from build123d import *

# Parameters (mm, degrees)
SKETCH1_W           = 45
SKETCH1_H           = 45
SKETCH1_R           = 1.55
SKETCH1_R_2         = 3.75
SKETCH1_R_3         = 1.5
BOSS_EXTRUDE2_DEPTH = 3
CHAMFER1_SIZE       = 2
FILLET2_R           = 10


with BuildPart() as part:
    # Sketch1 → Boss-Extrude2 (new body)
    # profile 1 of 3: a face of its own
    with BuildSketch(Plane(origin=(0, 0, 0), x_dir=(0, 0, -1), z_dir=(1, 0, 0))):
        Polygon((0, 15), (27.5, 86.038878339), (39.282646226, 75.31968933), (11.439152216, 14.16907058), (50, 14.16907058), (82.089729195, 14.16907058), (77.753857358, 26.374167507), (66.036256754, 25.688126343), (64.741637437, 39.196033454), (73.198877763, 39.196033454), (60.365916003, 75.31968933), (72.5, 85.972228566), (97.712949054, 15), (100, 15), (100, 0), (75, 0), (75, 10), (72, 10), (72, 0), (28, 0), (28, 10), (25, 10), (25, 0), (0, 0), align=None)
        with BuildLine():
            Line((67.956429084, 33.345444875), (77.753857358, 33.345444875))
            ThreePointArc((77.753857358, 33.345444875), (79.253857358, 31.845444875), (77.753857358, 30.345444875))
            Line((77.753857358, 30.345444875), (67.956429084, 30.345444875))
            ThreePointArc((67.956429084, 30.345444875), (66.456429084, 31.845444875), (67.956429084, 33.345444875))
        make_face(mode=Mode.SUBTRACT)
    # profile 2 of 3: a face of its own
    with BuildSketch(Plane(origin=(0, 0, 0), x_dir=(0, 0, -1), z_dir=(1, 0, 0))):
        with Locations((50, 97.81968933)):
            Rectangle(SKETCH1_W, SKETCH1_H)
        with Locations((34.5, 82.31968933)):
            Circle(SKETCH1_R, mode=Mode.SUBTRACT)
        with Locations((65.5, 82.31968933)):
            Circle(SKETCH1_R, mode=Mode.SUBTRACT)
        with Locations((65.5, 113.31968933)):
            Circle(SKETCH1_R, mode=Mode.SUBTRACT)
        with Locations((34.5, 113.31968933)):
            Circle(SKETCH1_R, mode=Mode.SUBTRACT)
        with Locations((50, 97.81968933)):
            Circle(SKETCH1_R_2, mode=Mode.SUBTRACT)
    # profile 3 of 3: a face of its own
    with BuildSketch(Plane(origin=(0, 0, 0), x_dir=(0, 0, -1), z_dir=(1, 0, 0))):
        Polygon((58.527688318, 120.31968933), (90.14613276, 143.005488448), (95.440133744, 135.626948458), (68.383623973, 116.214274737), align=None)
        with Locations((89.319967142, 136.74442097)):
            Circle(SKETCH1_R_3, mode=Mode.SUBTRACT)
    extrude(amount=BOSS_EXTRUDE2_DEPTH)

    # Chamfer1
    chamfer1_edges = [part.edges().sort_by_distance(p)[0] for p in [
        (3, 82.31968933, -32.95),
        (3, 113.31968933, -32.95),
        (3, 113.31968933, -63.95),
        (3, 82.31968933, -63.95),
    ]]
    chamfer(chamfer1_edges, length=CHAMFER1_SIZE)

    # Fillet2
    fillet2_edges = [part.edges().sort_by_distance(p)[0] for p in [
        (1.5, 86.038878339, -27.5),
        (1.5, 75.31968933, -60.365916003),
        (1.5, 75.31968933, -39.282646226),
    ]]
    fillet(fillet2_edges, radius=FILLET2_R)


solid = part.part
Here's how the part is built. I have some questions about the finished solid (model axes, mm). A direction names the side the tool comes from. Coordinates: 2 decimals unless noted, no trailing zeros. Order: outer loops, then holes, each group sorted by start corner. A loop starts at its lowest first (then second) coordinate and runs counter-clockwise, first axis right, second up. Notation, with made-up numbers: (72, 15.5) - (104, 15.5) arc R3 ccw to (104, 20.5) - close; hole circle Ø7 at (56, 34). An arc over 180 degrees is marked (long way). Use CSV: the item, a comma, the result in double quotes. Start each with the question number.
1. For faces 4 (the face through (3, 73, -62)), 5 (the face through (1, 5, -72)), 6 (the face through (1, 30.345, -73)), which set-ups out of +Z, -Z, +X, -X, +Y, -Y let a thin tool reach every point of the face, with its end or its side?
2. Suppose I cut it at B-B on y = 55.5. List the corners of the cut face in (x, z) for me, then the cut area to 3 significant figures.
3. Suppose I cut it at A-A on z = -50. List the corners of the cut face in (x, y) for me, then the cut area to 3 significant figures.
4. Suppose I cut it at D-D on z = -34.5. List the corners of the cut face in (x, y) for me, then the cut area to 3 significant figures.
5. If we mould it in two halves opening along Y, with no side actions, what happens to faces 1 (the face through (1, 10, -27)), 2 (the face through (1, 102, -72.5)), 3 (the face through (0, 73, -62))? For each: +Y half, -Y half, draft (parallel to the pull), parting line (faces both ways), or undercut.
6. Please list where these lines run through material, in increasing order: line 1 (Y direction, x = 2.2, z = -50); line 2 (Z direction, x = 2.35, y = 111); line 3 (Y direction, x = 1.5, z = -35.5). Write a range as from..to.
7. I'm going to push flat-ended pins straight in: pin 1 (12 mm diameter, centred on y = 68, z = -13.5, fed in from +X); pin 2 (3.5 mm diameter, centred on y = 82.32, z = -34.5, fed in from +X); pin 3 (1.5 mm diameter, centred on x = 1.5, z = -73, fed in from -Y). Where does each tip first touch, or does it pass through?
8. Suppose I cut it at C-C on z = -85.5. List the corners of the cut face in (x, y) for me.
Output:
1,face 4,"+Z, -Z, +X, +Y, -Y"
1,face 5,"+X, -X, -Y"
1,face 6,"+X, -X"
2,outline,"(0, -83.33) - (3, -83.33) - (3, -67.41) - (0, -67.41) - close; (0, -30.26) - (3, -30.26) - (3, -15.68) - (0, -15.68) - close"
2,area,"91.5 mm2"
3,outline,"(0, 0) - (3, 0) - (3, 14.17) - (0, 14.17) - close; (0, 75.32) - (3, 75.32) - (3, 94.07) - (0, 94.07) - close; (0, 101.57) - (3, 101.57) - (3, 120.32) - (0, 120.32) - close"
3,area,"155 mm2"
4,outline,"(0, 0) - (3, 0) - (3, 14.17) - (0, 14.17) - close; (0, 64.82) - (3, 64.82) - (3, 78.77) - (1, 80.77) - (0, 80.77) - close; (0, 83.87) - (1, 83.87) - (3, 85.87) - (3, 109.77) - (1, 111.77) - (0, 111.77) - close; (0, 114.87) - (1, 114.87) - (3, 116.87) - (3, 120.32) - (0, 120.32) - close"
4,area,"182 mm2"
5,face 1,"-Y half"
5,face 2,"undercut"
5,face 3,"draft"
6,line 1,"y = 0..14.17, 75.32..94.07, 101.57..120.32"
6,line 2,"z = -72.5..-67.24, -63.76..-36.24, -32.76..-27.5"
6,line 3,"y = 0..14.17, 67.01..80.53, 84.11..111.53, 115.11..120.32"
7,pin 1,"passes through"
7,pin 2,"stops at x = 1.2"
7,pin 3,"stops at y = 10"
8,outline,"(0, 0) - (3, 0) - (3, 49.38) - (0, 49.38) - close; (0, 128.5) - (3, 128.5) - (3, 139.67) - (0, 139.67) - close"
